Geometry: final body of the model. Coordinates: model frame, mm. A direction names the side the tool comes from. Coordinates: 2 decimals unless noted, no trailing zeros. Order: outer loops, then holes, each group sorted by start corner. A loop starts at its lowest first (then second) coordinate and runs counter-clockwise, first axis right, second up. Notation, with made-up numbers: M 39,-3.5 L 45,-3.5 A19 ccw 45,29.5 Z; hole C -37.5,-12.75 d3. An arc over 180 degrees is marked long. Use CSV: the item, a comma, the result in double quotes. Start each with the question number.
1. Material intervals for line 1 (Z direction, x = -3.5, y = 5); line 2 (Y direction, x = 21.5, z = 5.25); line 3 (X direction, y = 19, z = 2.25), sorted ascending.
2. Set-up query: faces 1 (the flat face through (47, 0, 3)), 2 (the flat face through (-1, 26, 3)). Return all of +Z, -Z, +X, -X, +Y, -Y with unobstructed straight access to the full face (end or side cutting, diameter ignored); none if empty.
3. Section query C-C on y = 13. Return the cut outline in (x, z).
4. Section query B-B on z = 4.5. Return the cut outline in (x, y).
5. Section query A-A on x = -12.5. Return the cut outline in (y, z), and give its area (3 significant figures).
6. Pull-direction query (Z, two-part tool) for faces 3 (the flat face through (-1, 0, 7)), 4 (the flat face through (-47, -2.1, 0.6)), 5 (the flat face through (-1, 0, 1)); classes: pulls with the +Z half, pulls with the -Z half, needs draft (parallel to the pull), parting line crosses it, or undercut.
from build123d import *

# Parameters (mm, degrees)
F1_W     = 94
F1_H     = 54
F2_DEPTH = 7
F3_W     = 52
F3_H     = 5
F4_DEPTH = 93


with BuildPart() as f2:
    # F1 (on Top) → F2 (new body)
    with BuildSketch(Plane.XY):
        Rectangle(F1_W, F1_H)
    extrude(amount=F2_DEPTH)

    # F3 (on face) → F4 (cut, through all)
    with BuildSketch(Plane(origin=(-47, 0, 0), x_dir=(0, -1, 0), z_dir=(-1, 0, 0))):
        with Locations((0, 3.5)):
            Rectangle(F3_W, F3_H)
    extrude(amount=-F4_DEPTH, mode=Mode.SUBTRACT)


solid = f2.part
Results list:
1,line 1,"z = 0 to 1, 6 to 7"
1,line 2,"y = -27 to -26, 26 to 27"
1,line 3,"x = 46 to 47"
2,face 1,"+Z, -Z, +X, +Y, -Y"
2,face 2,"-X"
3,outline,"M -47,0 L 47,0 L 47,7 L -47,7 L -47,6 L 46,6 L 46,1 L -47,1 Z"
4,outline,"M -47,-27 L 47,-27 L 47,27 L -47,27 L -47,26 L 46,26 L 46,-26 L -47,-26 Z"
5,outline,"M -27,0 L 27,0 L 27,7 L -27,7 Z; hole M -26,1 L 26,1 L 26,6 L -26,6 Z"
5,area,"118 mm²"
6,face 3,"pulls with the +Z half"
6,face 4,"needs draft"
6,face 5,"undercut"
